```python
from build123d import *

# Parameters (mm, degrees)
SKETCH3_R               = 90
BOSS_EXTRUDE1_DEPTH     = 210
BOSS_EXTRUDE2_DEPTH     = 50
BOSS_EXTRUDE3_DEPTH     = 210
SKETCH4_R               = 123
CUT_EXTRUDE1_DEPTH      = 25
CUT_EXTRUDE2_START      = -30
CUT_EXTRUDE2_DEPTH      = 30
CUT_EXTRUDE3_DEPTH      = 402.528330258
CUT_EXTRUDE3_DEPTH_BACK = 402.528330258
SKETCH8_R               = 2.5
SKETCH9_R               = 37.5
CUT_EXTRUDE4_DEPTH      = 1
SKETCH10_R              = 5
BOSS_EXTRUDE4_DEPTH     = 8
SKETCH11_R              = 13.401847331
BOSS_EXTRUDE5_DEPTH     = 4


with BuildPart() as part:
    # Sketch3 → Boss-Extrude1 (new body)
    with BuildSketch(Plane(origin=(0, 0, 0), x_dir=(1, 0, 0), z_dir=(0, 1, 0))):
        with Locations(Location((220, 0, 0), (0, 0, 270))):
            Circle(SKETCH3_R)
    extrude(amount=BOSS_EXTRUDE1_DEPTH)

    # Sketch3_3 → Boss-Extrude2 (add)
    with BuildSketch(Plane(origin=(0, 0, 0), x_dir=(1, 0, 0), z_dir=(0, 1, 0))):
        with BuildLine():
            ThreePointArc((-125.288461538, -34.681427383), (-78.71281484, -103.461552182), (0, -130))
            Line((0, -130), (220, -94))
            Line((220, -94), (220, -90))
            ThreePointArc((220, -90), (130, 0), (220, 90))
            Line((220, 90), (220, 94))
            Line((220, 94), (0, 130))
            ThreePointArc((0, 130), (-78.71281484, 103.461552182), (-125.288461538, 34.681427383))
            ThreePointArc((-125.288461538, 34.681427383), (-130, 0), (-125.288461538, -34.681427383))
        make_face()
    extrude(amount=BOSS_EXTRUDE2_DEPTH)

    # Sketch3_4 → Boss-Extrude3 (add)
    with BuildSketch(Plane(origin=(0, 0, 0), x_dir=(1, 0, 0), z_dir=(0, 1, 0))):
        with BuildLine():
            ThreePointArc((-125.288461538, 34.681427383), (-165, 0), (-125.288461538, -34.681427383))
            ThreePointArc((-125.288461538, -34.681427383), (-130, 0), (-125.288461538, 34.681427383))
        make_face()
    extrude(amount=BOSS_EXTRUDE3_DEPTH)

    # Sketch4 → Cut-Extrude1 (cut)
    with BuildSketch(Plane(origin=(0, 50, 0), x_dir=(1, 0, 0), z_dir=(0, 1, 0))):
        with Locations(Location((0, 0, 0), (0, 0, 270))):
            Circle(SKETCH4_R)
    extrude(amount=-CUT_EXTRUDE1_DEPTH, mode=Mode.SUBTRACT)

    # Sketch6 → Cut-Extrude2 (cut)
    with BuildSketch(Plane(origin=(0, 210, 0), x_dir=(1, 0, 0), z_dir=(0, 1, 0)).offset(CUT_EXTRUDE2_START)):
        with BuildLine():
            Line((-161.622776602, 15), (-129.131715701, 15))
            ThreePointArc((-129.131715701, 15), (-130, 0), (-129.131715701, -15))
            Line((-129.131715701, -15), (-161.622776602, -15))
            ThreePointArc((-161.622776602, -15), (-165, 0), (-161.622776602, 15))
        make_face()
    extrude(amount=CUT_EXTRUDE2_DEPTH, mode=Mode.SUBTRACT)

    # Sketch8 → Cut-Extrude3 (cut, two sides: drawn at the far end of the back side and taken through both)
    with BuildSketch(Plane(origin=(0, 0, 15), x_dir=(-1, 0, 0), z_dir=(0, 0, -1)).offset(-CUT_EXTRUDE3_DEPTH_BACK)):
        with Locations((149.131715701, 195)):
            Circle(SKETCH8_R)
    extrude(amount=CUT_EXTRUDE3_DEPTH + CUT_EXTRUDE3_DEPTH_BACK, mode=Mode.SUBTRACT)

    # Sketch9 → Cut-Extrude4 (cut)
    with BuildSketch(Plane(origin=(0, 25, 0), x_dir=(1, 0, 0), z_dir=(0, 1, 0))):
        with Locations(Location((0, 0, 0), (0, 0, 270))):
            Circle(SKETCH9_R)
    extrude(amount=-CUT_EXTRUDE4_DEPTH, mode=Mode.SUBTRACT)

    # Sketch10 → Boss-Extrude4 (add)
    with BuildSketch(Plane(origin=(0, 24, 0), x_dir=(1, 0, 0), z_dir=(0, 1, 0))):
        with Locations(Location((0, 0, 0), (0, 0, 270))):
            Circle(SKETCH10_R)
    extrude(amount=BOSS_EXTRUDE4_DEPTH)

    # Sketch11 → Boss-Extrude5 (add)
    with BuildSketch(Plane(origin=(0, 50, 0), x_dir=(1, 0, 0), z_dir=(0, 1, 0))):
        with Locations(Location((133.690962694, -79.625060242, 0), (0, 0, 270))):
            Circle(SKETCH11_R)
    extrude(amount=BOSS_EXTRUDE5_DEPTH)


solid = part.part
```
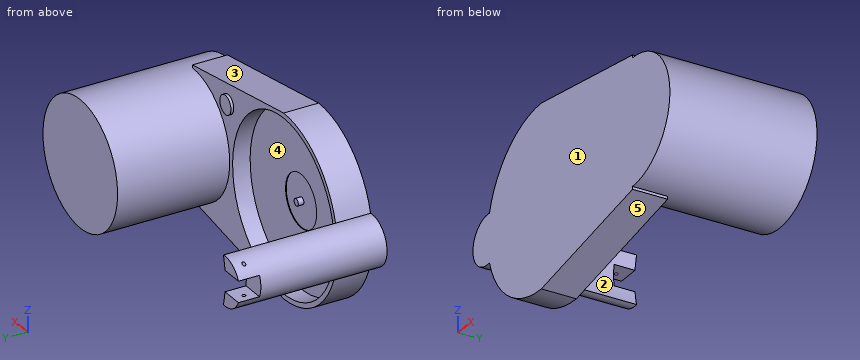
Could you check a few things on this model? Use its own coordinates, in mm. Face numbers are marked on the shaded views. A direction names the side the tool comes from. Give positions to 0.01 mm unless a question says otherwise; leave off trailing zeros. Order: outer loops, then holes, each group sorted by start corner. A loop starts at its lowest first (then second) coordinate and runs counter-clockwise, first axis right, second up.
Q1. Suppose I cut it at B-B, the plane z = 0. Write out the boundary of the cut face in (x, y).
Q2. If I drill on line 1 along X through (y, z) = (24.6, 0); line 2 along X through (y, z) = (195, -23); line 3 along Y through (x, z) = (-1.5, 100), over which ranges is the centre line in solid material (lowest first)?
Q3. Suppose I cut it at A-A, the plane y = 186.5. Write out the boundary of the cut face in (x, z).
Q4. We'd pull the mould along Z, two halves only. Please class the marked faces 3, 4 and 5: +Z half, -Z half, draft (parallel to the pull), parting line (faces both ways), or undercut.
Q5. Suppose I cut it at D-D, the plane x = -56. Write out the boundary of the cut face in (y, z).
Q6. I'm going to push flat-ended pins straight in: P1, Ø21.5, axis at x = 139, z = 78.5, coming from the +Y side; P2, Ø9, axis at x = -150.5, z = -1.5, coming from the +Y side; P3, Ø1.5, axis at x = -97.5, z = -83, coming from the +Y side. Where does each tip first touch, or does it pass through?
Q7. For the marked faces 1 and 2, which set-ups out of +Z, -Z, +X, -X, +Y, -Y let a thin tool reach every point of the face, with its end or its side?
Q8. Suppose I cut it at C-C, the plane x = 174. Write out the boundary of the cut face in (y, z), and give its area (3 significant figures).
Solution:
1. outline: (-165, 0) - (310, 0) - (310, 210) - (130, 210) - (130, 50) - (123, 50) - (123, 25) - (37.5, 25) - (37.5, 24) - (5, 24) - (5, 32) - (-5, 32) - (-5, 24) - (-37.5, 24) - (-37.5, 25) - (-123, 25) - (-123, 50) - (-130, 50) - (-130, 180) - (-165, 180) - close
2. line 1: x = -165 to -37.5, -5 to 5, 37.5 to 310
2. line 2: x = -156.38 to -151.63, -146.63 to -127.95, 132.99 to 307.01
2. line 3: y = 0 to 25
3. outline: (-161.62, -15) arc R35 ccw to (-125.29, -34.68) arc R130 cw to (-129.13, -15) - close; (-161.62, 15) - (-129.13, 15) arc R130 cw to (-125.29, 34.68) arc R35 ccw to start; circle Ø180 at (220, 0)
4. face 3: +Z half
4. face 4: undercut
4. face 5: -Z half
5. outline: (0, -117.32) - (50, -117.32) - (50, -109.51) - (25, -109.51) - (25, 109.51) - (50, 109.51) - (50, 117.32) - (0, 117.32) - close
6. P1: stops at y = 54
6. P2: stops at y = 180
6. P3: stops at y = 50
7. face 1: +Z, -Z, +X, -X, -Y
7. face 2: +Y
8. outline: (0, -101.53) - (50, -101.53) - (50, -77.36) - (210, -77.36) - (210, 77.36) - (50, 77.36) - (50, 101.53) - (0, 101.53) - close
8. area: 34,900 mm2
